CAD build for the part. Positions are in the model's coordinates, mm. Give positions to 0.01 mm unless a question says otherwise; leave off trailing zeros. Write each loop counter-clockwise with the first axis right and the second up, starting at its lowest first coordinate (ties: lowest second). Pieces come first, ordered by that corner, then holes. Notation, with made-up numbers: (64.25, -10.5) - (77.25, -10.5) arc R18 cw to (77.25, 21.5) - close; hole circle Ø1 at (55, -32). An arc over 180 degrees is marked (long way). Answer as a JSON object with one key per item and string values.
from build123d import *

# Parameters (mm, degrees)
SKETCH_1_R      = 30
SKETCH_1_R_2    = 2
SKETCH_1_R_3    = 3
EXTRUDE_1_DEPTH = 10


with BuildPart() as part:
    # 草图1 → 凸台-拉伸1 (new body)
    with BuildSketch(Plane(origin=(0, 0, 0), x_dir=(0, 0, -1), z_dir=(1, 0, 0))):
        with Locations((-12.848392551, 0.04812132)):
            Circle(SKETCH_1_R)
        with Locations((-12.848392551, 17.29812132)):
            Circle(SKETCH_1_R_2, mode=Mode.SUBTRACT)
        with Locations((2.090545664, 8.67312132)):
            Circle(SKETCH_1_R_2, mode=Mode.SUBTRACT)
        with Locations((2.090545664, -8.57687868)):
            Circle(SKETCH_1_R_2, mode=Mode.SUBTRACT)
        with Locations((-12.848392551, -17.20187868)):
            Circle(SKETCH_1_R_2, mode=Mode.SUBTRACT)
        with Locations((-27.787330766, -8.57687868)):
            Circle(SKETCH_1_R_2, mode=Mode.SUBTRACT)
        with Locations((-27.787330766, 8.67312132)):
            Circle(SKETCH_1_R_2, mode=Mode.SUBTRACT)
        with Locations((-12.848392551, 25.04812132)):
            Circle(SKETCH_1_R_3, mode=Mode.SUBTRACT)
        with Locations((12.151607449, 0.04812132)):
            Circle(SKETCH_1_R_3, mode=Mode.SUBTRACT)
        with Locations((-12.848392551, -24.95187868)):
            Circle(SKETCH_1_R_3, mode=Mode.SUBTRACT)
        with Locations((-37.848392551, 0.04812132)):
            Circle(SKETCH_1_R_3, mode=Mode.SUBTRACT)
    extrude(amount=EXTRUDE_1_DEPTH)


solid = part.part
(1) Saw through at A-A, the plane z = 14. Give the cut face in (x, y).
Answer key:
{"outline": "(0, -29.93) - (10, -29.93) - (10, -27.72) - (0, -27.72) - close; (0, -22.18) - (10, -22.18) - (10, -18.84) - (0, -18.84) - close; (0, -15.57) - (10, -15.57) - (10, 15.66) - (0, 15.66) - close; (0, 18.93) - (10, 18.93) - (10, 22.28) - (0, 22.28) - close; (0, 27.82) - (10, 27.82) - (10, 30.03) - (0, 30.03) - close"}
(2) Probe L1, parallel to Y at x = 2, z = 29.5; L2, parallel to Y at x = 7, z = 27.5; L3, parallel to Z at x = 4.25, y = 2. List the from-to ranges inside material, lowest first. Write a range as [from, to].
Answer key:
{"L1": "y = [-24.91, -9.61], [-7.54, 7.64], [9.71, 25]", "L2": "y = [-26.13, -10.56], [-6.6, 6.69], [10.65, 26.23]", "L3": "z = [-17.09, -14.43], [-9.87, 35.57], [40.13, 42.78]"}
(3) Flat gauge pins, fed straight in: P1, Ø1, axis at x = 8, y = -19.5, coming from the +Z side; P2, Ø1.5, axis at x = 4, y = -20.5, coming from the -Z side; P3, Ø3, axis at x = 6, y = -23.5, coming from the -Z side. Where does each tip first touch, or does it go through?
Answer key:
{"P1": "stops at z = 36.03", "P2": "stops at z = -9.69", "P3": "stops at z = -7.5"}
(4) Pull direction Y, two halves, no side cores. Call faces 1 (the face through (10, 0, 13)), 2 (the face through (4.93, 0.18, 40.845)), 3 (the face through (4.93, -29.24, 19.35)): pulls with the +Y half, pulls with the -Y half, needs draft (parallel to the pull), parting line crosses it, or undercut.
Answer key:
{"face 1": "needs draft", "face 2": "undercut", "face 3": "parting line crosses it"}
(5) Saw through at D-D, the plane y = -11.5. Give the cut face in (x, z).
Answer key:
{"outline": "(0, -14.84) - (10, -14.84) - (10, 40.54) - (0, 40.54) - close"}
(6) Saw through at B-B, the plane z = 26.5. Give the cut face in (x, y).
Answer key:
{"outline": "(0, -26.67) - (10, -26.67) - (10, -10.11) - (0, -10.11) - close; (0, -7.05) - (10, -7.05) - (10, 7.14) - (0, 7.14) - close; (0, 10.2) - (10, 10.2) - (10, 26.76) - (0, 26.76) - close"}
(7) Saw through at C-C, the plane x = 8. State how many separate pieces and enclosed holes the cut face has, and give its area (3 significant figures).
Answer key:
{"separate pieces": "1", "enclosed holes": "10", "area": "2,640 mm²"}
